Source: CAD feature listing. Evaluate the final solid. Frame: model axes, mm. Round coordinates to 2 decimals unless told otherwise and drop trailing zeros. Loops run counter-clockwise (first coordinate to the right, second up) from the corner with the lowest first, then second, coordinate; pieces in that order, holes last.
Item 1: Section query D-D on x = 23. Return loops of the section in (y, z).
Item 2: Ray query, L1, parallel to Y at x = 56, z = 0.4; L2, parallel to Y at x = 55.5, z = 1.6; L3, parallel to X at y = -7.5, z = 0.55. Return the intervals inside material, ascending.
Item 3: First-contact query: P1, Ø1.2, axis at x = 38.5, z = 1.5, coming from the -Y side; P2, Ø0.8, axis at x = 54.5, z = 1, coming from the +Y side; P3, Ø1.5, axis at x = 25, z = 2.5, coming from the +Y side. Flat tips, straight axial feed; report the tip coordinate or a pass-through.
Item 4: Section query B-B on y = -35. Return loops of the section in (x, z).
Item 5: Section query C-C on z = 1.8. Give the number of separate pieces and of enclosed holes in the cut face, then the cut area to 3 significant figures.
Item 6: Section query A-A on y = -12. Return loops of the section in (x, z), then the cut area to 3 significant figures.
```python
from build123d import *

# Parameters (mm, degrees)
SKETCH1_W           = 90
SKETCH1_H           = 90
BOSS_EXTRUDE5_DEPTH = 3
FILLET14_R          = 5
FILLET15_R          = 5
SKETCH17_R          = 10
SKETCH17_R_2        = 2
SKETCH17_W          = 7.5
SKETCH17_H          = 6
SKETCH17_W_2        = 6
SKETCH17_H_2        = 10
CUT_EXTRUDE4_DEPTH  = 3
FILLET16_R          = 0.5


with BuildPart() as part:
    # Sketch1 → Boss-Extrude5 (new body)
    with BuildSketch(Plane.XY):
        with Locations((55.696781823, -9)):
            Rectangle(SKETCH1_W, SKETCH1_H)
    extrude(amount=BOSS_EXTRUDE5_DEPTH)

    # Fillet14
    fillet14_edges = [part.edges().sort_by_distance(p)[0] for p in [
        (10.696781823, 36, 1.5),
        (100.696781823, 36, 1.5),
        (100.696781823, -54, 1.5),
        (10.696781823, -54, 1.5),
    ]]
    fillet(fillet14_edges, radius=FILLET14_R)

    # Fillet15
    # the kernel refuses this fillet: 5 mm, written as the material it takes off along each edge
    with BuildSketch(Plane(origin=(15.696781823, 31, 3), x_dir=(0, 1, 0), z_dir=(1, 0, 0))) as fillet15_piece_1:
        with BuildLine():
            CenterArc((0.417424305, -5), FILLET15_R, 23.578178478, 66.421821522)
            Line((0.417424305, 0), (0.417424305, 0.1))
            Line((0.417424305, 0.1), (5, 0.1))
            Line((5, 0.1), (5.1, 0))
            ThreePointArc((5.1, 0), (5.1, -1.5), (5.091651514, -2.96))
            Line((5.091651514, -2.96), (5, -3))
        make_face()
    revolve(axis=Axis((15.696781823, 31, 3), (0, 0, 1)), revolution_arc=90, mode=Mode.SUBTRACT)
    with BuildSketch(Plane(origin=(15.696781823, 36, 3), x_dir=(0, 0, -1), z_dir=(1, 0, 0))) as fillet15_piece_2:
        with BuildLine():
            CenterArc((5, -4.582575695), FILLET15_R, 113.578178478, 66.421821522)
            Line((0, -4.582575695), (-0.1, -4.582575695))
            Line((-0.1, -4.582575695), (-0.1, 0))
            Line((-0.1, 0), (0, 0.1))
            ThreePointArc((0, 0.1), (1.5, 0.1), (2.96, 0.091651514))
            Line((2.96, 0.091651514), (3, 0))
        make_face()
    extrude(amount=80, mode=Mode.SUBTRACT)
    with BuildSketch(Plane(origin=(95.696781823, 31, 3), x_dir=(0, 1, 0), z_dir=(-1, 0, 0))) as fillet15_piece_3:
        with BuildLine():
            CenterArc((0.417424305, 5), FILLET15_R, 270, 66.421821522)
            Line((0.417424305, 0), (0.417424305, -0.1))
            Line((0.417424305, -0.1), (5, -0.1))
            Line((5, -0.1), (5.1, 0))
            ThreePointArc((5.1, 0), (5.1, 1.5), (5.091651514, 2.96))
            Line((5.091651514, 2.96), (5, 3))
        make_face()
    revolve(axis=Axis((95.696781823, 31, 3), (0, 0, -1)), revolution_arc=90, mode=Mode.SUBTRACT)
    with BuildSketch(Plane(origin=(100.696781823, 31, 3), x_dir=(-1, 0, 0), z_dir=(0, -1, 0)), Plane(origin=(95.696781823, -54, 3), x_dir=(0, 1, 0), z_dir=(-1, 0, 0)), Plane(origin=(10.696781823, -49, 3), x_dir=(1, 0, 0), z_dir=(0, 1, 0))) as fillet15_piece_4:
        with BuildLine():
            CenterArc((4.582575695, 5), FILLET15_R, 203.578178478, 66.421821522)
            Line((0, 3), (-0.091651514, 2.96))
            ThreePointArc((-0.091651514, 2.96), (-0.1, 1.5), (-0.1, 0))
            Line((-0.1, 0), (0, -0.1))
            Line((0, -0.1), (4.582575695, -0.1))
            Line((4.582575695, -0.1), (4.582575695, 0))
        make_face()
    extrude(amount=80, mode=Mode.SUBTRACT)
    with BuildSketch(Plane(origin=(95.696781823, -49, 3), x_dir=(1, 0, 0), z_dir=(0, 1, 0))) as fillet15_piece_5:
        with BuildLine():
            CenterArc((0.417424305, 5), FILLET15_R, 270, 66.421821522)
            Line((5, 3), (5.091651514, 2.96))
            ThreePointArc((5.091651514, 2.96), (5.1, 1.5), (5.1, 0))
            Line((5.1, 0), (5, -0.1))
            Line((5, -0.1), (0.417424305, -0.1))
            Line((0.417424305, -0.1), (0.417424305, 0))
        make_face()
    revolve(axis=Axis((95.696781823, -49, 3), (0, 0, -1)), revolution_arc=90, mode=Mode.SUBTRACT)
    with BuildSketch(Plane(origin=(15.696781823, -49, 3), x_dir=(0, -1, 0), z_dir=(1, 0, 0))) as fillet15_piece_6:
        with BuildLine():
            CenterArc((0.417424305, 5), FILLET15_R, 270, 66.421821522)
            Line((5, 3), (5.091651514, 2.96))
            ThreePointArc((5.091651514, 2.96), (5.1, 1.5), (5.1, 0))
            Line((5.1, 0), (5, -0.1))
            Line((5, -0.1), (0.417424305, -0.1))
            Line((0.417424305, -0.1), (0.417424305, 0))
        make_face()
    revolve(axis=Axis((15.696781823, -49, 3), (0, 0, -1)), revolution_arc=90, mode=Mode.SUBTRACT)

    # Sketch17 → Cut-Extrude4 (cut)
    with BuildSketch(Plane.XY.offset(3)):
        with Locations((77.551683104, 13.009941811)):
            Circle(SKETCH17_R)
        with Locations((18.19937678, -7.407199345)):
            Circle(SKETCH17_R_2)
        with Locations((93.263694242, -7.407199345)):
            Circle(SKETCH17_R_2)
        with Locations((69.739484947, -34.653171103)):
            Rectangle(SKETCH17_W, SKETCH17_H)
        with Locations((55.687795517, -8.716286613)):
            Rectangle(SKETCH17_W_2, SKETCH17_H_2)
        with Locations((40.465326937, -34.674989483)):
            Rectangle(SKETCH17_W, SKETCH17_H)
        with BuildLine():
            Line((53.707261797, 6.745948723), (57.423415647, 6.745948723))
            ThreePointArc((57.423415647, 6.745948723), (58.423415647, 5.745948723), (57.423415647, 4.745948723))
            Line((57.423415647, 4.745948723), (53.707261797, 4.745948723))
            ThreePointArc((53.707261797, 4.745948723), (52.707261797, 5.745948723), (53.707261797, 6.745948723))
        make_face()
        with BuildLine():
            Line((51.807146289, 15.44525347), (58.394003545, 15.44525347))
            ThreePointArc((58.394003545, 15.44525347), (60.894003545, 12.94525347), (58.394003545, 10.44525347))
            Line((58.394003545, 10.44525347), (51.807146289, 10.44525347))
            ThreePointArc((51.807146289, 10.44525347), (49.307146289, 12.94525347), (51.807146289, 15.44525347))
        make_face()
    extrude(amount=-CUT_EXTRUDE4_DEPTH, mode=Mode.SUBTRACT)

    # Fillet16
    fillet16_edges = [part.edges().sort_by_distance(p)[0] for p in [
        (16.19937678, -7.407199345, 3),
        (91.263694242, -7.407199345, 3),
        (52.687795517, -8.716286613, 3),
        (55.687795517, -13.716286613, 3),
        (58.687795517, -8.716286613, 3),
        (55.687795517, -3.716286613, 3),
        (36.715326937, -34.674989483, 3),
        (40.465326937, -37.674989483, 3),
        (44.215326937, -34.674989483, 3),
        (40.465326937, -31.674989483, 3),
        (65.989484947, -34.653171103, 3),
        (69.739484947, -37.653171103, 3),
        (73.489484947, -34.653171103, 3),
        (69.739484947, -31.653171103, 3),
    ]]
    fillet(fillet16_edges, radius=FILLET16_R)


solid = part.part
```
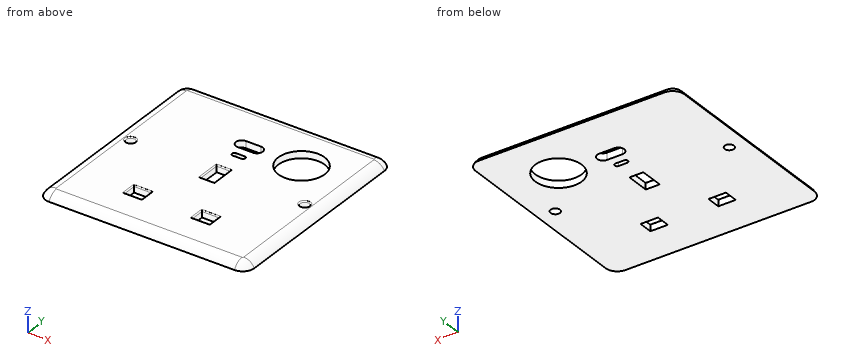
Data:
1. outline: (-54, 0) - (36, 0) arc R5 ccw to (31.42, 3) - (-49.42, 3) arc R5 ccw to start
2. L1: y = -53.8 to -13.72, -3.72 to 4.75, 6.75 to 10.45, 15.45 to 35.8
2. L2: y = -52.89 to -13.72, -3.72 to 4.75, 6.75 to 10.45, 15.45 to 34.89
2. L3: x = 10.98 to 16.2, 20.2 to 52.69, 58.69 to 91.27, 95.26 to 100.42
3. P1: stops at y = -53.49
3. P2: stops at y = 35.69
3. P3: stops at y = 34.72
4. outline: (10.7, 0) - (36.72, 0) - (36.72, 2.5) arc R0.5 ccw to (36.22, 3) - (15.28, 3) arc R5 ccw to start; (44.22, 0) - (65.99, 0) - (65.99, 2.5) arc R0.5 ccw to (65.49, 3) - (44.72, 3) arc R0.5 ccw to (44.22, 2.5) - close; (73.49, 0) - (100.7, 0) arc R5 ccw to (96.11, 3) - (73.99, 3) arc R0.5 ccw to (73.49, 2.5) - close
5. separate pieces: 1
5. enclosed holes: 8
5. area: 7,060 mm2
6. outline: (10.7, 0) - (52.69, 0) - (52.69, 2.5) arc R0.5 ccw to (52.19, 3) - (15.28, 3) arc R5 ccw to start; (58.69, 0) - (100.7, 0) arc R5 ccw to (96.11, 3) - (59.19, 3) arc R0.5 ccw to (58.69, 2.5) - close
6. area: 244 mm2
